from build123d import *

# Parameters (mm, degrees)
SKETCH1_W           = 109.99978
SKETCH1_H           = 109.99978
BOSS_EXTRUDE1_DEPTH = 9.525
SKETCH2_R           = 5.9055
CUT_EXTRUDE1_DEPTH  = 5.5118
SKETCH3_R           = 2.7305
CUT_EXTRUDE3_DEPTH  = 10.525
SKETCH4_R           = 4.2545
CUT_EXTRUDE4_DEPTH  = 10.525
FILLET1_R           = 9.525


with BuildPart() as part:
    # Sketch1 → Boss-Extrude1 (new body)
    with BuildSketch(Plane.XY):
        Rectangle(SKETCH1_W, SKETCH1_H)
    extrude(amount=-BOSS_EXTRUDE1_DEPTH)

    # Sketch2 → Cut-Extrude1 (cut)
    with BuildSketch(Plane.XY):
        with Locations((45.06849, 1.06299)):
            Circle(SKETCH2_R)
        with Locations((-45.06849, 1.06299)):
            Circle(SKETCH2_R)
        with BuildLine():
            Line((-29.7053, 27.05989), (29.7053, 27.05989))
            ThreePointArc((29.7053, 27.05989), (35.6108, 21.15439), (29.7053, 15.24889))
            Line((29.7053, 15.24889), (-29.7053, 15.24889))
            ThreePointArc((-29.7053, 15.24889), (-35.6108, 21.15439), (-29.7053, 27.05989))
        make_face()
        with BuildLine():
            Line((-5.9055, -0.8255), (-5.9055, -38.9255))
            ThreePointArc((-5.9055, -38.9255), (0, -44.831), (5.9055, -38.9255))
            Line((5.9055, -38.9255), (5.9055, -0.8255))
            ThreePointArc((5.9055, -0.8255), (0, 5.08), (-5.9055, -0.8255))
        make_face()
        with BuildLine():
            Line((20.32, -13.12291), (40.64, -13.12291))
            ThreePointArc((40.64, -13.12291), (46.5455, -19.02841), (40.64, -24.93391))
            Line((40.64, -24.93391), (20.32, -24.93391))
            ThreePointArc((20.32, -24.93391), (14.4145, -19.02841), (20.32, -13.12291))
        make_face()
        with BuildLine():
            Line((-20.32, -13.12291), (-40.64, -13.12291))
            ThreePointArc((-40.64, -13.12291), (-46.5455, -19.02841), (-40.64, -24.93391))
            Line((-40.64, -24.93391), (-20.32, -24.93391))
            ThreePointArc((-20.32, -24.93391), (-14.4145, -19.02841), (-20.32, -13.12291))
        make_face()
    extrude(amount=-CUT_EXTRUDE1_DEPTH, mode=Mode.SUBTRACT)

    # Sketch3 → Cut-Extrude3 (cut, through all)
    with BuildSketch(Plane.XY):
        with BuildLine():
            ThreePointArc((29.7053, 23.88489), (32.4358, 21.15439), (29.7053, 18.42389))
            Line((29.7053, 18.42389), (-29.7053, 18.42389))
            ThreePointArc((-29.7053, 18.42389), (-32.4358, 21.15439), (-29.7053, 23.88489))
            Line((-29.7053, 23.88489), (29.7053, 23.88489))
        make_face()
        with BuildLine():
            Line((3.048, -0.8255), (2.7305, -38.9255))
            ThreePointArc((2.7305, -38.9255), (0, -41.656), (-2.7305, -38.9255))
            Line((-2.7305, -38.9255), (-3.048, -0.8255))
            ThreePointArc((-3.048, -0.8255), (0, 2.2225), (3.048, -0.8255))
        make_face()
        with BuildLine():
            Line((-20.32, -16.29791), (-40.64, -16.29791))
            ThreePointArc((-40.64, -16.29791), (-43.3705, -19.02841), (-40.64, -21.75891))
            Line((-40.64, -21.75891), (-20.32, -21.75891))
            ThreePointArc((-20.32, -21.75891), (-17.5895, -19.02841), (-20.32, -16.29791))
        make_face()
        with BuildLine():
            ThreePointArc((40.64, -16.29791), (43.3705, -19.02841), (40.64, -21.75891))
            Line((40.64, -21.75891), (20.32, -21.75891))
            ThreePointArc((20.32, -21.75891), (17.5895, -19.02841), (20.32, -16.29791))
            Line((20.32, -16.29791), (40.64, -16.29791))
        make_face()
        with Locations((-45.06849, 1.06299)):
            Circle(SKETCH3_R)
        with Locations((45.06849, 1.06299)):
            Circle(SKETCH3_R)
    extrude(amount=-CUT_EXTRUDE3_DEPTH, mode=Mode.SUBTRACT)

    # Sketch4 → Cut-Extrude4 (cut, through all)
    with BuildSketch(Plane.XY):
        with Locations((-39.99865, -39.99865)):
            Circle(SKETCH4_R)
        with Locations((-39.99865, 39.99865)):
            Circle(SKETCH4_R)
        with Locations((39.99865, -39.99865)):
            Circle(SKETCH4_R)
        with Locations((39.99865, 39.99865)):
            Circle(SKETCH4_R)
    extrude(amount=-CUT_EXTRUDE4_DEPTH, mode=Mode.SUBTRACT)

    # Fillet1
    fillet1_edges = [part.edges().sort_by_distance(p)[0] for p in [
        (-54.99989, 54.99989, -4.7625),
        (-54.99989, -54.99989, -4.7625),
        (54.99989, -54.99989, -4.7625),
        (54.99989, 54.99989, -4.7625),
    ]]
    fillet(fillet1_edges, radius=FILLET1_R)


solid = part.part
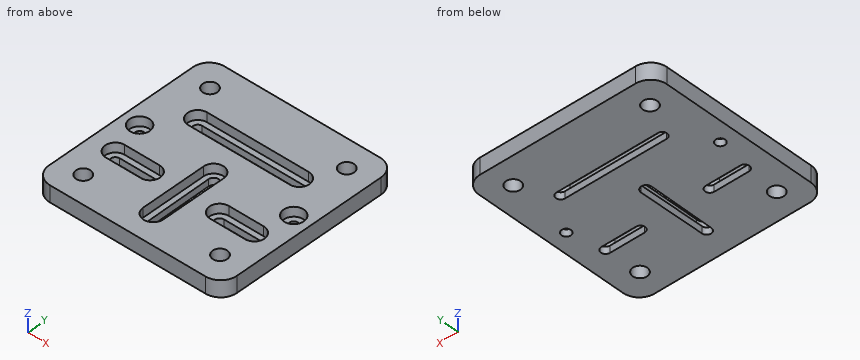
Can you work these out from the model? Positions are in its coordinate system, mm. Round coordinates to 2 decimals unless told otherwise and drop trailing zeros. Order: outer loops, then holes, each group sorted by start corner. A loop starts at its lowest first (then second) coordinate and runs counter-clockwise, first axis right, second up. Notation, with made-up numbers: M 14,-31 L 22,-31 A33 cw 22,-1 Z; hole C -20,47.5 d4. An arc over 180 degrees is marked long. Use a Markdown table: item, result.
1) Imagine slicing it at A-A (x = 0). List the corners of the cut face in (y, z) for me (1 decimal).
Geometry says:
| item | result |
|---|---|
| outline | M -55,-9.5 L -41.7,-9.5 L -41.7,-5.5 L -44.8,-5.5 L -44.8,0 L -55,0 Z; M 2.2,-9.5 L 18.4,-9.5 L 18.4,-5.5 L 15.2,-5.5 L 15.2,0 L 5.1,0 L 5.1,-5.5 L 2.2,-5.5 Z; M 23.9,-9.5 L 55,-9.5 L 55,0 L 27.1,0 L 27.1,-5.5 L 23.9,-5.5 Z |
2) I'm going to push a flat-ended pin straight in: P1, Ø6, axis at x = -1.5, y = -19.5, coming from the +Z side. Where does the tip first touch, or does it pass through?
Geometry says:
| item | result |
|---|---|
| P1 | stops at z = -5.51 |
3) If I drill on line 1 along Y through (x, z) = (22, -6.25); line 2 along Y through (x, z) = (26.5, -3); line 3 along X through (y, z) = (-30, -1.25), over which ranges is the centre line in solid material (lowest first)?
Geometry says:
| item | result |
|---|---|
| line 1 | y = -55 to -21.76, -16.3 to 18.42, 23.88 to 55 |
| line 2 | y = -55 to -24.93, -13.12 to 15.25, 27.06 to 55 |
| line 3 | x = -55 to -5.91, 5.91 to 55 |
4) Imagine slicing it at B-B (y = -20.5). List the corners of the cut face in (x, z) for me (1 decimal).
Geometry says:
| item | result |
|---|---|
| outline | M -55,-9.5 L -42.9,-9.5 L -42.9,-5.5 L -46.4,-5.5 L -46.4,0 L -55,0 Z; M -18,-9.5 L -2.9,-9.5 L -2.9,-5.5 L -5.9,-5.5 L -5.9,0 L -14.6,0 L -14.6,-5.5 L -18,-5.5 Z; M 2.9,-9.5 L 18,-9.5 L 18,-5.5 L 14.6,-5.5 L 14.6,0 L 5.9,0 L 5.9,-5.5 L 2.9,-5.5 Z; M 42.9,-9.5 L 55,-9.5 L 55,0 L 46.4,0 L 46.4,-5.5 L 42.9,-5.5 Z |
5) Imagine slicing it at D-D (x = -25). List the corners of the cut face in (y, z) for me (3 decimals).
Geometry says:
| item | result |
|---|---|
| outline | M -55,-9.525 L -21.759,-9.525 L -21.759,-5.512 L -24.934,-5.512 L -24.934,0 L -55,0 Z; M -16.298,-9.525 L 18.424,-9.525 L 18.424,-5.512 L 15.249,-5.512 L 15.249,0 L -13.123,0 L -13.123,-5.512 L -16.298,-5.512 Z; M 23.885,-9.525 L 55,-9.525 L 55,0 L 27.06,0 L 27.06,-5.512 L 23.885,-5.512 Z |
6) Imagine slicing it at C-C (z = -3.75). Give the number of separate pieces and of enclosed holes in the cut face, then the cut area to 3 significant figures.
Geometry says:
| item | result |
|---|---|
| separate pieces | 1 |
| enclosed holes | 10 |
| area | 9,510 mm² |
